Could you check a few things on this model? Use its own coordinates, in mm. Face numbers are marked on the shaded views. A direction names the side the tool comes from. Round coordinates to 2 decimals unless told otherwise and drop trailing zeros. Write each loop counter-clockwise with the first axis right and the second up, starting at its lowest first coordinate (ties: lowest second). Pieces come first, ordered by that corner, then holes. Notation, with made-up numbers: (74, -30) - (87, -30) arc R18 ccw to (87, -6) - close; hole circle Ø2 at (79.25, 18). An arc over 180 degrees is marked (long way). Write each question's results on one line, items separated by ' | '. Start each with the question number.
(1) Imagine slicing it at D-D on z = -0.5. Write out the boundary of the cut face in (x, y).
(2) For P1, Ø1.6, axis at y = -4.5, z = 1, coming from the -X side; P2, Ø1, axis at y = -4.5, z = 1, coming from the +X side; P3, Ø3, axis at x = -4, z = 1, coming from the -Y side, each with a flat end and sliding along its axis, tell me the tip position at first contact or that it passes through.
(3) Thinking about a two-plate mould opening in X: for the marked faces 3, 4 and 5, which applies, +X half, -X half, draft (parallel to the pull), parting line (faces both ways), or undercut?
(4) Please list where these lines run through material, in increasing order: line 1 (X direction, y = -5.75, z = 0.7); line 2 (Z direction, x = -1.5, y = -6.25); line 3 (Y direction, x = 5, z = 1.15). Write a range as [from, to].
(5) Imagine slicing it at B-B on z = 0.5. Write out the boundary of the cut face in (x, y).
(6) Imagine slicing it at A-A on x = 0. Write out the boundary of the cut face in (y, z), then the cut area to 3 significant figures.
(7) Imagine slicing it at C-C on y = -4.75. Write out the boundary of the cut face in (x, z), then the cut area to 3 significant figures.
(8) On a 3-axis mill with a long thin cutter (end or side, diameter ignored), from which of +Z, -Z, +X, -X, +Y, -Y can I reach the whole of each face in a straight line? I mean the marked faces 1 and 2. Say none if no direction works.
```python
from build123d import *
from build123d import SkipClean  # not in build123d's __all__

# Parameters (mm, degrees)
F1_R     = 7.45
F2_DEPTH = 3.4
F3_DEPTH = 2


with BuildPart() as f2:
    # F1 (on Top) → F2 (new body)
    with BuildSketch(Plane.XY):
        Circle(F1_R)
    extrude(amount=-F2_DEPTH)

    # F0 (on Top) → F3 (join)
    with BuildSketch(Plane.XY):
        with BuildLine():
            Line((2.25, -6.5), (2.25, -7.1021123618))
            ThreePointArc((2.25, -7.1021123618), (0, 7.45), (-2.25, -7.1021123618))
            Line((-2.25, -7.1021123618), (-2.25, -6.5))
            Line((-2.25, -6.5), (-2.25, -3.5))
            Line((-2.25, -3.5), (2.25, -3.5))
            Line((2.25, -3.5), (2.25, -6.5))
        make_face()
    with SkipClean():  # cleaning this boolean's faces spoils the solid; the shape is the same uncleaned
        extrude(amount=F3_DEPTH)


solid = f2.part
```
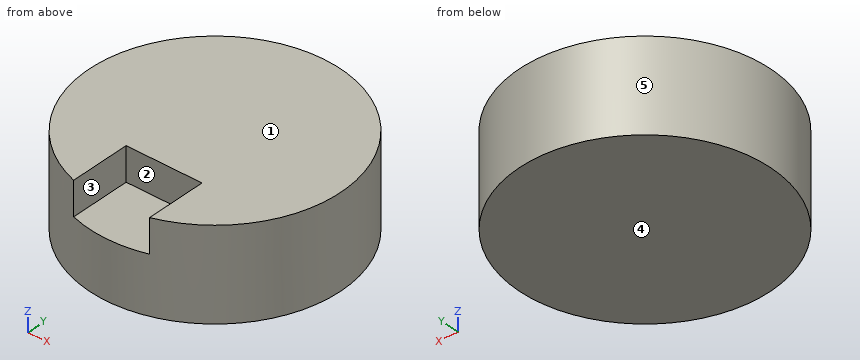
Response:
1) outline: circle Ø14.9 at (0, 0)
2) P1: x = -6.47 | P2: x = 6.29 | P3: y = -7.02
3) face 3: undercut | face 4: draft | face 5: parting line
4) line 1: [-4.74, -2.25], [2.25, 4.74] | line 2: [-3.4, 0] | line 3: [-5.52, 5.52]
5) outline: (-2.25, -7.1) - (-2.25, -3.5) - (2.25, -3.5) - (2.25, -7.1) arc R7.45 ccw (long way) to start
6) outline: (-7.45, -3.4) - (7.45, -3.4) - (7.45, 2) - (-3.5, 2) - (-3.5, 0) - (-7.45, 0) - close | area: 72.6 mm²
7) outline: (-5.74, -3.4) - (5.74, -3.4) - (5.74, 2) - (2.25, 2) - (2.25, 0) - (-2.25, 0) - (-2.25, 2) - (-5.74, 2) - close | area: 53.0 mm²
8) face 1: +Z, +X, -X, +Y, -Y | face 2: +Z, -Y
